The listing builds one solid part. Answer for the finished solid, in the listing's coordinates (mm). Face numbers are marked on the shaded views. Give positions to 0.01 mm unless a question says otherwise; leave off trailing zeros. Loops run counter-clockwise (first coordinate to the right, second up) from the corner with the lowest first, then second, coordinate; pieces in that order, holes last.
Item 1: Consider line 1 along Z through (x, y) = (-14.4, 0); line 2 along Y through (x, z) = (3, 59); line 3 along Z through (x, y) = (-8, 0). Determine where each line is inside the solid, lowest interval first.
Item 2: Each of these flat-tipped pins is pushed along its axis until it touches: pin 1 Ø8 at (x, z) = (-3, 102.5) entering from -Y; pin 2 Ø4 at (x, y) = (5.5, 24.5) entering from +Z; pin 3 Ø5 at (x, y) = (8, -72.5) entering from +Z. Where does it stop, or does it pass through?
Item 3: The mould has two halves that part along Y. Classify the marked faces 1, 2 and 3: pulls with the +Y half, pulls with the -Y half, needs draft (parallel to the pull), parting line crosses it, or undercut.
Item 4: Section A-A, the plane y = 0 is taken. Give the vertices of the cut face in (x, z).
Item 5: Section B-B, the plane x = -4.5 is taken. Give the vertices of the cut face in (y, z).
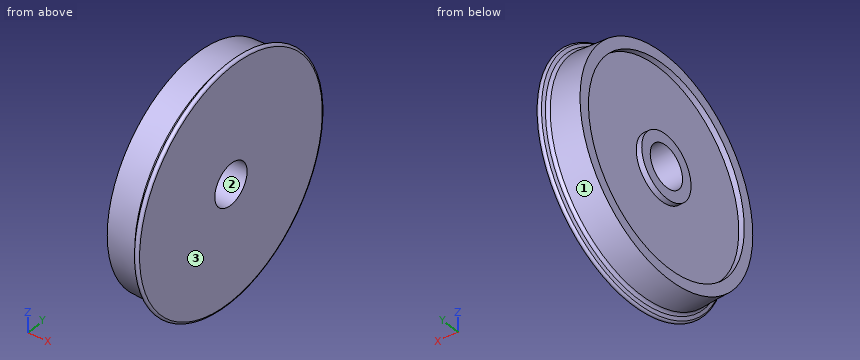
from build123d import *


with BuildPart() as f1:
    # F0 (on Front) → F1 (revolve)
    with BuildSketch(Plane.XZ):
        with BuildLine():
            Line((-17, -41.921168), (-17, -51.921168))
            Line((-17, -51.921168), (9.06, -53.286915))
            ThreePointArc((9.06, -53.286915), (10.785108, -53.906292), (11.881794, -55.374933))
            Line((11.881794, -55.374933), (13.004233, -58.458809))
            ThreePointArc((13.004233, -58.458809), (15.297715, -59.782951), (17, -57.754247))
            Line((17, -57.754247), (17, -51.921168))
            Line((17, -51.921168), (17, 30.678832))
            Line((17, 30.678832), (-17, 30.678832))
            Line((-17, 30.678832), (-17, 20.678832))
            Line((-17, 20.678832), (-12, 20.678832))
            Line((-12, 20.678832), (-12, -41.921168))
            Line((-12, -41.921168), (-17, -41.921168))
        make_face()
    revolve(axis=Axis((0, 0, 49.678832), (-1, 0, 0)))


solid = f1.part
Worked answers:
1. line 1: z = -52.06 to -41.92, 20.68 to 30.68, 68.68 to 78.68, 141.28 to 151.42
1. line 2: y = -102.22 to -16.56, 16.56 to 102.22
1. line 3: z = -52.39 to 30.68, 68.68 to 151.75
2. pin 1: stops at y = -89.95
2. pin 2: stops at z = 149.98
2. pin 3: stops at z = 125.12
3. face 1: parting line crosses it
3. face 2: undercut
3. face 3: needs draft
4. outline: (-17, -51.92) - (9.06, -53.29) arc R3.18 cw to (11.88, -55.37) - (13, -58.46) arc R2.06 ccw to (17, -57.75) - (17, 30.68) - (-17, 30.68) - (-17, 20.68) - (-12, 20.68) - (-12, -41.92) - (-17, -41.92) - close; (-17, 68.68) - (17, 68.68) - (17, 157.11) arc R2.06 ccw to (13, 157.82) - (11.88, 154.73) arc R3.18 cw to (9.06, 152.64) - (-17, 151.28) - (-17, 141.28) - (-12, 141.28) - (-12, 78.68) - (-17, 78.68) - close
5. outline: circle Ø204.51 at (0, 49.68); hole circle Ø38 at (0, 49.68)
